Autodesk Inventor part; units mm, degrees
ref_plane "YZ Plane" through (0, 0, 0) normal (1, 0, 0) x (0, 1, 0)
ref_plane "XZ Plane" through (0, 0, 0) normal (0, 1, 0) x (-1, 0, 0)
ref_plane "XY Plane" through (0, 0, 0) normal (0, 0, 1) x (1, 0, 0)
sketch "Sketch1" plane through (0, 0, 0) normal (0, 1, 0) x (-1, 0, 0)
  line L0 (20, -15.715) -> (-20, -15.715)
  line L1 (-20, -15.715) -> (-20, 15.715)
  line L2 (-20, 15.715) -> (20, 15.715)
  line L3 (20, 15.715) -> (20, -15.715)
  point P0 (0, 0)
  dimension "d0" = 40
  dimension "d1" = 20
  dimension "d2" = 31.43
  dimension "d3" = 15.715
extrude "Plate1" add sketch "Sketch1" along normal blind 1.5
sketch "Sketch2" plane through (20, 0, 17.215) normal (0, 0, -1) x (-1, 0, 0)
  line L0 (40, 0) -> (0, 0)
  line L1 (0, 0) -> (0, 45)
  line L2 (0, 45) -> (40, 45)
  line L3 (40, 45) -> (40, 0)
edge flange "Flange1" height 45 angle 90 thickness 1.5 bend radius 0.31 thickness toward (0, 0, -1) relief tear relief width 1.5 relief depth 0.75 edges at (0, 1.5, 15.715) wall of the first edge with corners at (-20, 0, 17.215) (20, 0, 17.215) (20, 45, 17.215) (-20, 45, 17.215)
bend "Bend1"
corner "Corner1"
sketch "Sketch3" plane through (-20, 0, -17.215) normal (0, 0, 1) x (1, 0, 0)
  line L0 (40, 0) -> (0, 0)
  line L1 (0, 0) -> (0, 45)
  line L2 (0, 45) -> (40, 45)
  line L3 (40, 45) -> (40, 0)
edge flange "Flange2" height 45 angle 90 thickness 1.5 bend radius 0.31 thickness toward (0, 0, 1) relief tear relief width 1.5 relief depth 0.75 edges at (0, 1.5, -15.715) wall of the first edge with corners at (20, 0, -17.215) (-20, 0, -17.215) (-20, 45, -17.215) (20, 45, -17.215)
bend "Bend2"
corner "Corner2"
sketch "Sketch4" plane through (-20, 45, 17.215) normal (0, 0, 1) x (1, 0, 0)
  line L0 (0, -43.19) -> (0, 0)
  line L1 (0, 0) -> (40, 0)
  line L2 (40, 0) -> (40, -43.19)
  line L3 (0, -43.19) -> (40, -43.19)
  arc A0 (28.9876, -5.6156) -> (11.0124, -5.6156) centre (20, -10) ccw
  line L4 (0, -38.19) -> (40, -38.19)
  line L5 (40, -38.19) -> (40, -28.19)
  line L6 (40, -28.19) -> (0, -28.19)
  line L7 (0, -28.19) -> (0, -38.19)
  line L8 (40, -28.19) -> (28.9876, -5.6156)
  line L9 (11.0124, -5.6156) -> (0, -28.19)
  point P0 (0, -28.19)
  point P1 (20, 0)
  point P2 (40, -28.19)
  dimension "d50" = 10
  dimension "d51" = 20
  dimension "d52" = 20
  dimension "d53" = 38.19
  dimension "d54" = 10
  dimension "d55" = 40
  dimension "d56" = 40
extrude "Extrusion1" cut sketch "Sketch4" against normal blind 50 contours L0 L1 A0 L9 | L8 A0 L1 L2
sketch "Sketch6" plane through (-20, 1.81, 17.215) normal (0, 0, 1) x (1, 0, 0)
  arc A0 (28.9876, 37.5744) -> (11.0124, 37.5744) centre (20, 33.19) ccw
  point P0 (20, -1.81)
hole "Hole2" at (0, 35, 17.215) direction (0, 0, -1) diameter 5.1 depth 1.5
sketch "Sketch7" plane through (-20, 1.81, -15.715) normal (0, 0, 1) x (1, 0, 0)
  arc A0 (28.9876, 37.5744) -> (11.0124, 37.5744) centre (20, 33.19) ccw
  point P0 (20, -1.81)
hole "Hole3" at (0, 35, -15.715) direction (0, 0, -1) diameter 5.2 depth 1.5
sketch "Sketch8" plane through (0, 1.5, 0) normal (0, 1, 0) x (1, 0, 0)
  line L0 (20, 15.405) -> (20, -15.405)
  line L1 (20, -15.715) -> (-20, -15.715)
  line L2 (-20, -15.405) -> (20, -15.405)
  line L3 (20, 15.405) -> (-20, 15.405)
  point P0 (0, 0)
  point P1 (14, -9.405)
  point P2 (-14, -9.405)
  point P3 (14, 0)
  point P4 (-14, 0)
  point P5 (14, 9.405)
  point P6 (-14, 9.405)
  dimension "d71" = 6
  dimension "d73" = 6
  dimension "d76" = 28
  dimension "d79" = 9.405
hole "Hole4" at (14, 1.5, 9.405) at (-14, 1.5, 9.405) at (14, 1.5, 0) at (-14, 1.5, 0) at (14, 1.5, -9.405) at (-14, 1.5, -9.405) direction (0, -1, 0) diameter 2.1 depth 1.5
sketch "Sketch9" plane through (20, 1.81, -17.215) normal (0, 0, -1) x (-1, 0, 0)
  arc A0 (28.9876, 37.5744) -> (11.0124, 37.5744) centre (20, 33.19) ccw
  circle A1 centre (20, 40.19) radius 1.05
  circle A2 centre (13, 33.19) radius 1.05
  circle A3 centre (20, 26.19) radius 1.05
  circle A4 centre (27, 33.19) radius 1.05
  point P0 (20, -1.81)
  dimension "d89" = 7
  dimension "d90" = 0
  dimension "d91" = 2.1
  dimension "d94" = 360
hole "Hole5" at (0, 28, -17.215) at (7, 35, -17.215) at (-7, 35, -17.215) at (0, 42, -17.215) direction (0, 0, 1) diameter 2.1 depth 1.5
equation "\"d62\" = Thickness"
equation "\"d69\" = Thickness"
equation "\"d87\" = Thickness"
equation "\"d101\" = Thickness"
equation "\"d4\" = Thickness"
equation "\"d5\" = BendReliefWidth"
equation "\"d6\" = BendReliefDepth"
equation "\"d7\" = MinimumRemnant"
equation "\"d8\" = TransitionRadius"
equation "\"d11\" = BendRadius"
equation "\"d12\" = CornerReliefSize"
equation "\"d13\" = GapSize"
equation "\"d14\" = JacobiRadiusSize"
equation "\"d15\" = BendReliefWidth"
equation "\"d16\" = BendReliefDepth"
equation "\"d17\" = MinimumRemnant"
equation "\"d18\" = TransitionRadius"
equation "\"d21\" = BendRadius"
equation "\"d22\" = CornerReliefSize"
equation "\"d23\" = GapSize"
equation "\"d24\" = JacobiRadiusSize"
equation "\"BendReliefWidth\" = Thickness"
equation "\"BendReliefDepth\" = 0.5 * Thickness"
equation "\"CornerReliefSize\" = 4 * Thickness"
equation "\"MinimumRemnant\" = 2 * Thickness"
equation "\"TransitionRadius\" = BendRadius"
equation "\"JacobiRadiusSize\" = BendRadius"
equation "\"GapSize\" = Thickness"
properties part number "axis_12_bottom_frame(top)" material "Aluminum 6061-AHC"
CAD build for the part. Positions are in the model's coordinates, mm. A direction names the side the tool comes from. Round coordinates to 2 decimals unless told otherwise and drop trailing zeros. Write each loop counter-clockwise with the first axis right and the second up, starting at its lowest first coordinate (ties: lowest second). Pieces come first, ordered by that corner, then holes. Notation, with made-up numbers: (24.25, 18) - (56.25, 18) arc R17 cw to (56.25, 37) - close; hole circle Ø3 at (17, 17.25). An arc over 180 degrees is marked (long way). Return JSON: item names as keys, results as strings. Group by question number.
Item 1: Band-saw the part on C-C on y = 42. List the corners of the cut face in (x, z) (3 decimals), plus the area to 3 significant figures.
Item 2: Mould opens along Z. For faces 4 (the face through (14.57, 27.94, -16.45)), 5 (the face through (0, 18, 15.715)) say: +Z half, -Z half, draft (parallel to the pull), parting line (faces both ways), or undercut.
Item 3: Band-saw the part on A-A on y = 16. List the corners of the cut face in (x, z) (3 decimals), plus the area to 3 significant figures.
Item 4: Probe probe 1 along Z at (x, y) = (12.5, 26.5) (3 decimals); probe 2 along X at (y, z) = (35, -16.75); probe 3 along Y at (x, z) = (0, -16.65). List the from-to ranges inside material, lowest first.
Item 5: Flat gauge pins, fed straight in: pin 1 Ø15.5 at (x, z) = (-2, -6.5) entering from +Y; pin 2 Ø1.9 at (x, z) = (14, 0) entering from +Y. Where does each tip first touch, or does it go through?
Item 6: 3-axis set-ups, long thin cutter, end or side, ignore diameter. For faces 1 (the face through (0, 18, -15.715)), 2 (the face through (12.96, 0.74, -9.54)), 3 (the face through (-7.05, 33.95, -16.45)): which of +Z, -Z, +X, -X, +Y, -Y reach the whole face in a straight line?
Item 7: Band-saw the part on B-B on x = 0. List the corners of the cut face in (y, z) (3 decimals), plus the area to 3 significant figures.
Item 8: Band-saw the part on D-D on x = 14. List the corners of the cut face in (y, z) (3 decimals), plus the area to 3 significant figures.
Resolved:
{
 "1": {"outline": "(-7.141, -17.215) - (-1.05, -17.215) - (-1.05, -15.715) - (-7.141, -15.715) - close; (-7.141, 15.715) - (7.141, 15.715) - (7.141, 17.215) - (-7.141, 17.215) - close; (1.05, -17.215) - (7.141, -17.215) - (7.141, -15.715) - (1.05, -15.715) - close", "area": "39.7 mm²"},
 "2": {"face 4": "draft", "face 5": "undercut"},
 "3": {"outline": "(-20, -17.215) - (20, -17.215) - (20, -15.715) - (-20, -15.715) - close; (-20, 15.715) - (20, 15.715) - (20, 17.215) - (-20, 17.215) - close", "area": "120 mm²"},
 "4": {"probe 1": "z = -17.215 to -15.715, 15.715 to 17.215", "probe 2": "x = -11.13 to -8.05, -5.95 to -2.6, 2.6 to 5.95, 8.05 to 11.13", "probe 3": "y = 0.5 to 26.95, 29.05 to 32.4, 37.6 to 40.95, 43.05 to 45"},
 "5": {"pin 1": "stops at y = 1.5", "pin 2": "passes through"},
 "6": {"face 1": "+X, -X, +Y", "face 2": "+Y, -Y", "face 3": "-Z"},
 "7": {"outline": "(0, -15.405) arc R1.81 ccw to (1.81, -17.215) - (26.95, -17.215) - (26.95, -15.715) - (1.81, -15.715) arc R0.31 cw to (1.5, -15.405) - (1.5, 15.405) arc R0.31 cw to (1.81, 15.715) - (32.45, 15.715) - (32.45, 17.215) - (1.81, 17.215) arc R1.81 ccw to (0, 15.405) - close; (29.05, -17.215) - (32.4, -17.215) - (32.4, -15.715) - (29.05, -15.715) - close; (37.55, 15.715) - (45, 15.715) - (45, 17.215) - (37.55, 17.215) - close; (37.6, -17.215) - (40.95, -17.215) - (40.95, -15.715) - (37.6, -15.715) - close; (43.05, -17.215) - (45, -17.215) - (45, -15.715) - (43.05, -15.715) - close", "area": "159 mm²"},
 "8": {"outline": "(0, -15.405) arc R1.81 ccw to (1.81, -17.215) - (29.109, -17.215) - (29.109, -15.715) - (1.81, -15.715) arc R0.31 cw to (1.5, -15.405) - (1.5, -10.455) - (0, -10.455) - close; (0, -8.355) - (1.5, -8.355) - (1.5, -1.05) - (0, -1.05) - close; (0, 1.05) - (1.5, 1.05) - (1.5, 8.355) - (0, 8.355) - close; (0, 10.455) - (1.5, 10.455) - (1.5, 15.405) arc R0.31 cw to (1.81, 15.715) - (29.109, 15.715) - (29.109, 17.215) - (1.81, 17.215) arc R1.81 ccw to (0, 15.405) - close", "area": "124 mm²"}
}
